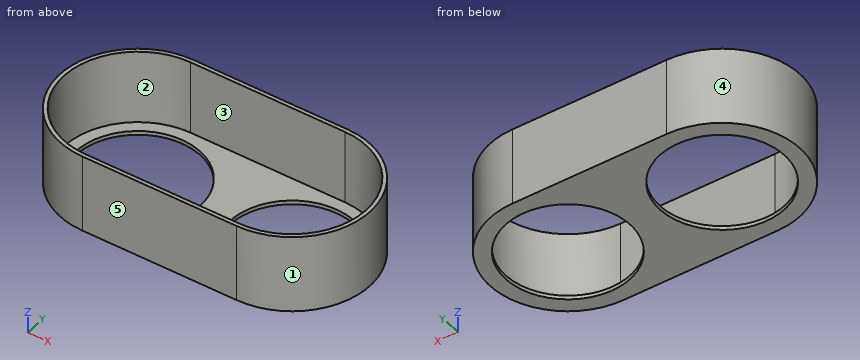
```python
from build123d import *

# Parameters (mm, degrees)
F1_DEPTH = 50
F2_T     = -2.5
F3_R     = 40
F4_DEPTH = 25


with BuildPart() as f1:
    # F0 (on Top) → F1 (new body)
    with BuildSketch(Plane.XY):
        with BuildLine():
            Line((50, 50), (-50, 50))
            ThreePointArc((-50, 50), (-100, 0), (-50, -50))
            Line((-50, -50), (50, -50))
            ThreePointArc((50, -50), (100, 0), (50, 50))
        make_face()
    extrude(amount=F1_DEPTH)

    # F2
    f2_openings = [f1.faces().sort_by_distance(p)[0] for p in [
        (0, 0, 50),
    ]]
    offset(amount=F2_T, openings=f2_openings)

    # F3 (on face) → F4 (cut)
    with BuildSketch(Plane.XY.offset(2.5)):
        with Locations((-50, 0)):
            Circle(F3_R)
        with Locations((50, 0)):
            Circle(F3_R)
    extrude(amount=-F4_DEPTH, mode=Mode.SUBTRACT)


solid = f1.part
```
Could you check a few things on this model? Use its own coordinates, in mm. Face numbers are marked on the shaded views. A direction names the side the tool comes from. Round coordinates to 2 decimals unless told otherwise and drop trailing zeros. Write each loop counter-clockwise with the first axis right and the second up, starting at its lowest first coordinate (ties: lowest second). Pieces come first, ordered by that corner, then holes. Notation, with made-up numbers: M 16,-9.75 L 45,-9.75 A18 cw 45,0.25 Z; hole C 49.25,-6.75 d11. An arc over 180 degrees is marked long. Answer in a Markdown table with one row per item. Add a question column.
Q1. If I drill on line 1 (Y direction, x = -39.5, z = 35); line 2 (Y direction, x = -50, z = 1.7); line 3 (X direction, y = 28, z = 2), over which ranges is the centre line in solid material (lowest first)? Write a range as from..to.
Q2. Imagine slicing it at B-B (y = 0). Please give me the cut outline in (x, z), then the cut area to 4 significant figures.
Q3. Imagine slicing it at A-A (x = -12). Please give me the cut outline in (y, z).
Q4. If we mould it in two halves opening along Y, with no side actions, what happens to the marked faces 3, 4 and 5? For each: +Y half, -Y half, draft (parallel to the pull), parting line (faces both ways), or undercut.
Q5. Imagine slicing it at C-C (z = 34). Please give me the cut outline in (x, y), then the cut area to 3 significant figures.
Q6. Will these pins go through, and if not, where does the flat tip stop? pin 1 Ø5 at (y, z) = (12.5, 36) entering from +X; pin 2 Ø2 at (x, y) = (18.5, 32.5) entering from -Z; pin 3 Ø4 at (y, z) = (37, 13.5) entering from -X; pin 4 Ø8 at (y, z) = (10.5, 35) entering from -X.
Q7. Imagine slicing it at D-D (y = 30.5). Please give me the cut outline in (x, z).
Q8. On a 3-axis mill with a long thin cutter (end or side, diameter ignored), from which of +Z, -Z, +X, -X, +Y, -Y can I reach the whole of each face in a straight line? I mean the marked faces 1 and 2. Say none if no direction works.
Values:
| question | item | result |
|---|---|---|
| 1 | line 1 | -50..-47.5, 47.5..50 |
| 1 | line 2 | -50..-40, 40..50 |
| 1 | line 3 | -91.42..-78.57, -21.43..21.43, 78.57..91.42 |
| 2 | outline | M -100,0 L -90,0 L -90,2.5 L -97.5,2.5 L -97.5,50 L -100,50 Z; M -10,0 L 10,0 L 10,2.5 L -10,2.5 Z; M 90,0 L 100,0 L 100,50 L 97.5,50 L 97.5,2.5 L 90,2.5 Z |
| 2 | area | 337.5 mm^2 |
| 3 | outline | M -50,0 L -12.49,0 L -12.49,2.5 L -47.5,2.5 L -47.5,50 L -50,50 Z; M 12.49,0 L 50,0 L 50,50 L 47.5,50 L 47.5,2.5 L 12.49,2.5 Z |
| 4 | face 3 | undercut |
| 4 | face 4 | parting line |
| 4 | face 5 | -Y half |
| 5 | outline | M -50,-50 L 50,-50 A50 ccw 50,50 L -50,50 A50 ccw Z; hole M -50,-47.5 L 50,-47.5 A47.5 ccw 50,47.5 L -50,47.5 A47.5 ccw Z |
| 5 | area | 1,270 mm^2 |
| 6 | pin 1 | x = 98.99 |
| 6 | pin 2 | z = 0 |
| 6 | pin 3 | x = -85.71 |
| 6 | pin 4 | x = -99.58 |
| 7 | outline | M -89.62,0 L -75.88,0 L -75.88,2.5 L -86.41,2.5 L -86.41,50 L -89.62,50 Z; M -24.12,0 L 24.12,0 L 24.12,2.5 L -24.12,2.5 Z; M 75.88,0 L 89.62,0 L 89.62,50 L 86.41,50 L 86.41,2.5 L 75.88,2.5 Z |
| 8 | face 1 | +Z, -Z, +X |
| 8 | face 2 | +Z |
